The figure shows three views and two pictorial views of one solid part (mm, origin at its lowest corner). Answer the questions. Give positions to 0.01 mm unless a question says otherwise; leave off trailing zeros. Order: outer loops, then holes, each group sorted by start corner. A loop starts at its lowest first (then second) coordinate and runs counter-clockwise, first axis right, second up. Notation, with made-up numbers: (80.25, -26.75) - (105.25, -26.75) arc R34 ccw to (105.25, 12.25) - close; hole circle Ø8 at (-33.75, -24). An arc over 180 degrees is marked (long way). Use a Markdown table: item, result. Add a question column.
1. A cutting plane is placed at C-C on y = 7. Determine the outline of the cut face in (x, z).
2. A cutting plane is placed at B-B on x = 30. Determine the outline of the cut face in (y, z).
3. For a pull along X with two mould halves and no side action, classify the marked faces 1, 2 and 3 as released by +X, released by -X, zero draft, split by the parting line, or undercut.
4. Flat-ended cylindrical pins translate along their axes: P1, Ø8, axis at x = 28, y = 9.5, coming from the -Z side; P2, Ø9.5, axis at x = 15, z = 77.5, coming from the +Y side; P3, Ø8, axis at x = 52, y = 12, coming from the -Z side. Find the tip coordinate at first contact, or state that the pin passes through.
5. A cutting plane is placed at A-A on z = 77.5. Determine the outline of the cut face in (x, y), and give its area (4 significant figures).
6. A cutting plane is placed at D-D on z = 13.5. Determine the outline of the cut face in (x, y), and give its area (3 significant figures).
7. Consider L1, parallel to X at y = 12, z = 77.5; L2, parallel to X at y = 23.6, z = 77.5; L3, parallel to Z at x = 17.5, y = 12.5. Determine where each line is inside the solid, lowest interval first.
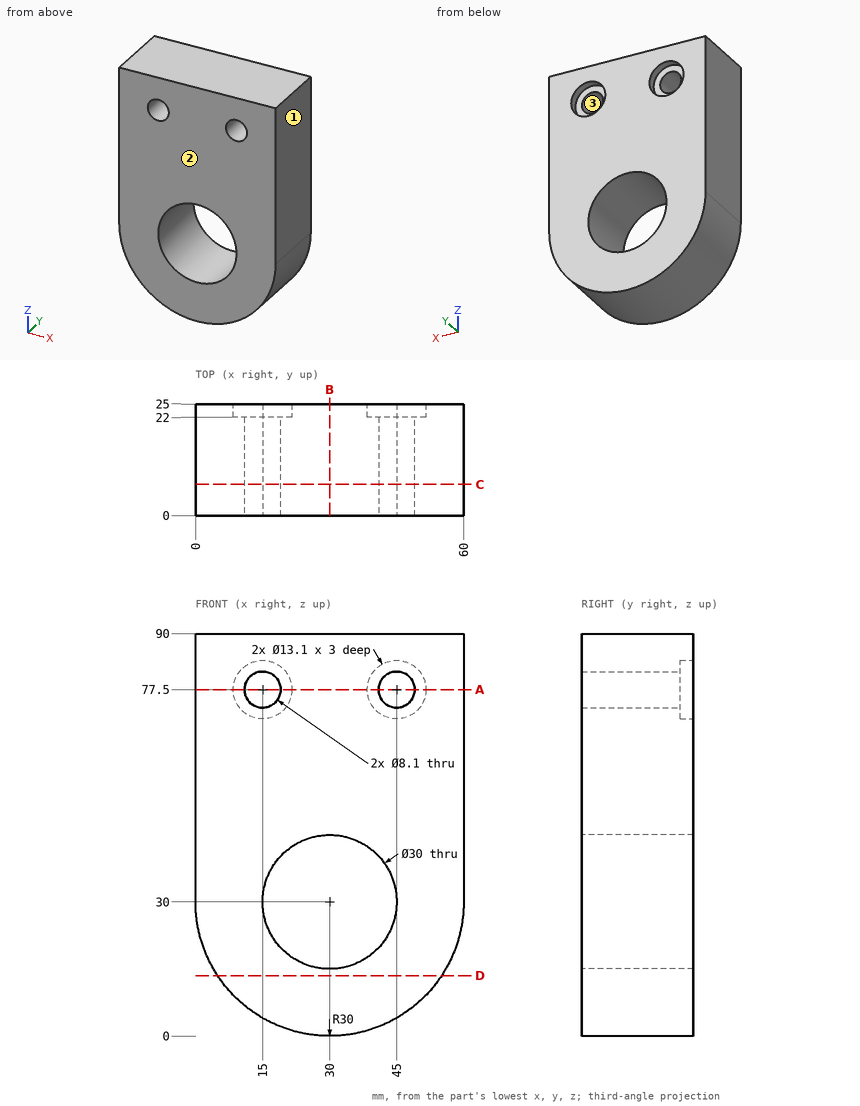
Output values:
| question | item | result |
|---|---|---|
| 1 | outline | (0, 30) arc R30 ccw to (60, 30) - (60, 90) - (0, 90) - close; hole circle Ø8.1 at (15, 77.5); hole circle Ø30 at (30, 30); hole circle Ø8.1 at (45, 77.5) |
| 2 | outline | (0, 0) - (25, 0) - (25, 15) - (0, 15) - close; (0, 45) - (25, 45) - (25, 90) - (0, 90) - close |
| 3 | face 1 | released by +X |
| 3 | face 2 | zero draft |
| 3 | face 3 | undercut |
| 4 | P1 | z = 0 |
| 4 | P2 | y = 22 |
| 4 | P3 | z = 6 |
| 5 | outline | (0, 0) - (10.95, 0) - (10.95, 22) - (8.45, 22) - (8.45, 25) - (0, 25) - close; (19.05, 0) - (40.95, 0) - (40.95, 22) - (38.45, 22) - (38.45, 25) - (21.55, 25) - (21.55, 22) - (19.05, 22) - close; (49.05, 0) - (60, 0) - (60, 25) - (51.55, 25) - (51.55, 22) - (49.05, 22) - close |
| 5 | area | 1,065 mm² |
| 6 | outline | (4.95, 0) - (55.05, 0) - (55.05, 25) - (4.95, 25) - close |
| 6 | area | 1,250 mm² |
| 7 | L1 | 0 to 10.95, 19.05 to 40.95, 49.05 to 60 |
| 7 | L2 | 0 to 8.45, 21.55 to 38.45, 51.55 to 60 |
| 7 | L3 | 2.73 to 21.71, 38.29 to 74.31, 80.69 to 90 |
